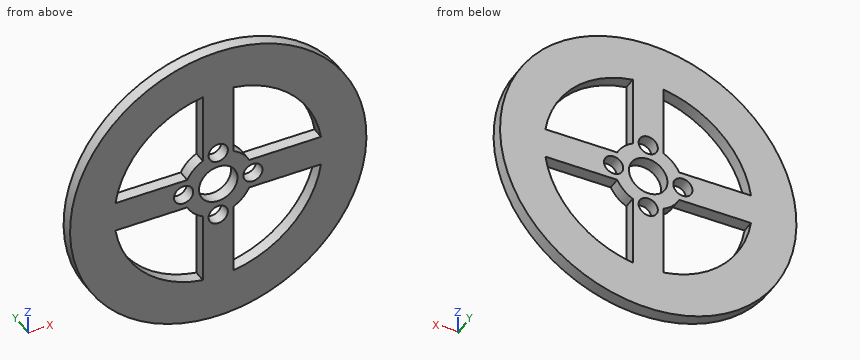
```python
from build123d import *

# Parameters (mm, degrees)
CROQUIS1_R              = 19.25
SALIENTE_EXTRUIR1_DEPTH = 1.6
CROQUIS2_R              = 2.5
CROQUIS2_R_2            = 1.25
CORTAR_EXTRUIR1_DEPTH   = 1.6
CORTAR_EXTRUIR2_DEPTH   = 1.6


with BuildPart() as part:
    # Croquis1 → Saliente-Extruir1 (new body)
    with BuildSketch(Plane(origin=(0, 0, 0), x_dir=(1, 0, 0), z_dir=(0, 1, 0))):
        with Locations(Location((0, 0, 0), (0, 0, 270))):
            Circle(CROQUIS1_R)
    extrude(amount=SALIENTE_EXTRUIR1_DEPTH)

    # Croquis2 → Cortar-Extruir1 (cut)
    with BuildSketch(Plane(origin=(0, 1.6, 0), x_dir=(1, 0, 0), z_dir=(0, 1, 0))):
        with Locations(Location((0, 0, 0), (0, 0, 270))):
            Circle(CROQUIS2_R)
        with Locations(Location((0, 4.5, 0), (0, 0, 270))):
            Circle(CROQUIS2_R_2)
        with Locations(Location((4.5, 0, 0), (0, 0, 270))):
            Circle(CROQUIS2_R_2)
        with Locations(Location((0, -4.5, 0), (0, 0, 270))):
            Circle(CROQUIS2_R_2)
        with Locations(Location((-4.5, 0, 0), (0, 0, 270))):
            Circle(CROQUIS2_R_2)
    extrude(amount=-CORTAR_EXTRUIR1_DEPTH, mode=Mode.SUBTRACT)

    # Croquis3 → Cortar-Extruir2 (cut)
    with BuildSketch(Plane(origin=(0, 1.6, 0), x_dir=(1, 0, 0), z_dir=(0, 1, 0))):
        with BuildLine():
            Line((-2, 4.031128874), (-2, 13.351029923))
            ThreePointArc((-2, 13.351029923), (-9.545941546, 9.545941546), (-13.351029923, 2))
            Line((-13.351029923, 2), (-4.031128874, 2))
            ThreePointArc((-4.031128874, 2), (-3.181980515, 3.181980515), (-2, 4.031128874))
        make_face()
        with BuildLine():
            ThreePointArc((13.351029923, 2), (9.545941546, 9.545941546), (2, 13.351029923))
            Line((2, 13.351029923), (2, 4.031128874))
            ThreePointArc((2, 4.031128874), (3.181980515, 3.181980515), (4.031128874, 2))
            Line((4.031128874, 2), (13.351029923, 2))
        make_face()
        with BuildLine():
            ThreePointArc((2, -13.351029923), (9.545941546, -9.545941546), (13.351029923, -2))
            Line((13.351029923, -2), (4.031128874, -2))
            ThreePointArc((4.031128874, -2), (3.181980515, -3.181980515), (2, -4.031128874))
            Line((2, -4.031128874), (2, -13.351029923))
        make_face()
        with BuildLine():
            Line((-4.031128874, -2), (-13.351029923, -2))
            ThreePointArc((-13.351029923, -2), (-9.545941546, -9.545941546), (-2, -13.351029923))
            Line((-2, -13.351029923), (-2, -4.031128874))
            ThreePointArc((-2, -4.031128874), (-3.181980515, -3.181980515), (-4.031128874, -2))
        make_face()
    extrude(amount=-CORTAR_EXTRUIR2_DEPTH, mode=Mode.SUBTRACT)


solid = part.part
```
Geometry: final body of the model. Coordinates: model frame, mm. Give positions to 0.01 mm unless a question says otherwise; leave off trailing zeros. Write each loop counter-clockwise with the first axis right and the second up, starting at its lowest first coordinate (ties: lowest second). Pieces come first, ordered by that corner, then holes.
1. Pin query (flat end, axial travel): P1, Ø0.5, axis at y = 0.5, z = 10.5, coming from the -X side; P2, Ø0.5, axis at x = 9, y = 1, coming from the -Z side; P3, Ø0.8, axis at y = 1, z = 7.5, coming from the +X side. Return the tip coordinate at first contact, or that it passes through.
2. Section query D-D, the plane x = -10. Return loops of the section in (y, z).
3. Section query C-C, the plane y = 0.9. Count the separate pieces of the cut face and the enclosed holes in it, then the cut area to 3 significant figures.
4. Section query A-A, the plane z = 0. Return loops of the section in (x, y), then the cut area to 3 significant figures.
5. Section query B-B, the plane x = 0. Return loops of the section in (y, z).
6. Line query: probe 1 along X at (y, z) = (0.95, 0); probe 2 along X at (y, z) = (1.5, -3.5); probe 3 along X at (y, z) = (1.5, 6). Output: solid intervals per line, ascending.
Computed:
1. P1: stops at x = -16.29
1. P2: stops at z = -17.15
1. P3: stops at x = 17.89
2. outline: (0, -16.45) - (1.6, -16.45) - (1.6, -9.07) - (0, -9.07) - close; (0, -2) - (1.6, -2) - (1.6, 2) - (0, 2) - close; (0, 9.07) - (1.6, 9.07) - (1.6, 16.45) - (0, 16.45) - close
3. separate pieces: 1
3. enclosed holes: 9
3. area: 762 mm2
4. outline: (-19.25, 0) - (-5.75, 0) - (-5.75, 1.6) - (-19.25, 1.6) - close; (-3.25, 0) - (-2.5, 0) - (-2.5, 1.6) - (-3.25, 1.6) - close; (2.5, 0) - (3.25, 0) - (3.25, 1.6) - (2.5, 1.6) - close; (5.75, 0) - (19.25, 0) - (19.25, 1.6) - (5.75, 1.6) - close
4. area: 45.6 mm2
5. outline: (0, -19.25) - (1.6, -19.25) - (1.6, -5.75) - (0, -5.75) - close; (0, -3.25) - (1.6, -3.25) - (1.6, -2.5) - (0, -2.5) - close; (0, 2.5) - (1.6, 2.5) - (1.6, 3.25) - (0, 3.25) - close; (0, 5.75) - (1.6, 5.75) - (1.6, 19.25) - (0, 19.25) - close
6. probe 1: x = -19.25 to -5.75, -3.25 to -2.5, 2.5 to 3.25, 5.75 to 19.25
6. probe 2: x = -18.93 to -13.04, -2.83 to -0.75, 0.75 to 2.83, 13.04 to 18.93
6. probe 3: x = -18.29 to -12.09, -2 to 2, 12.09 to 18.29
